from build123d import *

# Parameters (mm, degrees)
EXTRUDE1_DEPTH                                   = 7.9375
CBORE_FOR_1_4_SOCKET_HEAD_CAP_SCREW1_D           = 6.7564
CBORE_FOR_1_4_SOCKET_HEAD_CAP_SCREW1_DEPTH       = 9.525
CBORE_FOR_1_4_SOCKET_HEAD_CAP_SCREW1_CBORE_D     = 11.1125
CBORE_FOR_1_4_SOCKET_HEAD_CAP_SCREW1_CBORE_DEPTH = 6.35
F_1_4_20_TAPPED_HOLE1_D                          = 5.1054
CBORE_FOR_1_4_SOCKET_HEAD_CAP_SCREW2_D           = 6.7564
CBORE_FOR_1_4_SOCKET_HEAD_CAP_SCREW2_DEPTH       = 9.525
CBORE_FOR_1_4_SOCKET_HEAD_CAP_SCREW2_CBORE_D     = 11.1125
CBORE_FOR_1_4_SOCKET_HEAD_CAP_SCREW2_CBORE_DEPTH = 6.35
F_1_4_20_TAPPED_HOLE3_D                          = 5.1054
CBORE_FOR_1_4_SOCKET_HEAD_CAP_SCREW3_D           = 6.7564
CBORE_FOR_1_4_SOCKET_HEAD_CAP_SCREW3_DEPTH       = 9.525
CBORE_FOR_1_4_SOCKET_HEAD_CAP_SCREW3_CBORE_D     = 11.1125
CBORE_FOR_1_4_SOCKET_HEAD_CAP_SCREW3_CBORE_DEPTH = 6.35
F_1_4_20_TAPPED_HOLE4_D                          = 5.1054
FILLET1_R                                        = 3.175


with BuildPart() as part:
    # Sketch1 → Extrude1 (new, symmetric)
    with BuildSketch(Plane.XY):
        with BuildLine():
            Line((-39.6875, 82.55), (-39.6875, 0))
            ThreePointArc((-39.6875, 0), (-32.485618813, -22.798733003), (-13.49375, -37.323134477))
            Line((-13.49375, -37.323134477), (-13.49375, -56.373134477))
            Line((-13.49375, -56.373134477), (-3.96875, -56.373134477))
            Line((-3.96875, -56.373134477), (-3.96875, -36.296166184))
            ThreePointArc((-3.96875, -36.296166184), (0, 36.5125), (3.96875, -36.296166184))
            Line((3.96875, -36.296166184), (3.96875, -56.373134477))
            Line((3.96875, -56.373134477), (13.49375, -56.373134477))
            Line((13.49375, -56.373134477), (13.49375, -37.323134477))
            ThreePointArc((13.49375, -37.323134477), (32.485618813, -22.798733003), (39.6875, 0))
            Line((39.6875, 0), (39.6875, 31.75))
            Line((39.6875, 31.75), (58.7375, 31.75))
            Line((58.7375, 31.75), (58.7375, 41.275))
            Line((58.7375, 41.275), (-30.95625, 41.275))
            ThreePointArc((-30.95625, 41.275), (-34.925, 45.24375), (-30.95625, 49.2125))
            Line((-30.95625, 49.2125), (58.7375, 49.2125))
            Line((58.7375, 49.2125), (58.7375, 58.7375))
            Line((58.7375, 58.7375), (39.6875, 58.7375))
            Line((39.6875, 58.7375), (39.6875, 82.55))
            ThreePointArc((39.6875, 82.55), (32.485618813, 105.348733003), (13.49375, 119.873134477))
            Line((13.49375, 119.873134477), (13.49375, 138.923134477))
            Line((13.49375, 138.923134477), (3.96875, 138.923134477))
            Line((3.96875, 138.923134477), (3.96875, 110.719801693))
            ThreePointArc((3.96875, 110.719801693), (0, 54.102), (-3.96875, 110.719801693))
            Line((-3.96875, 110.719801693), (-3.96875, 138.923134477))
            Line((-3.96875, 138.923134477), (-13.49375, 138.923134477))
            Line((-13.49375, 138.923134477), (-13.49375, 119.873134477))
            ThreePointArc((-13.49375, 119.873134477), (-32.485618813, 105.348733003), (-39.6875, 82.55))
        make_face()
    extrude(amount=EXTRUDE1_DEPTH, both=True)

    # CBORE for 1/4 Socket Head Cap Screw1
    with Locations(Plane(origin=(13.49375, 0, 0), x_dir=(0, 0, -1), z_dir=(1, 0, 0))):
        with Locations((0, 129.398134477)):
            CounterBoreHole(CBORE_FOR_1_4_SOCKET_HEAD_CAP_SCREW1_D / 2, CBORE_FOR_1_4_SOCKET_HEAD_CAP_SCREW1_CBORE_D / 2, CBORE_FOR_1_4_SOCKET_HEAD_CAP_SCREW1_CBORE_DEPTH, depth=CBORE_FOR_1_4_SOCKET_HEAD_CAP_SCREW1_DEPTH)

    # 1/4-20 Tapped Hole1 (through all)
    with Locations(Plane(origin=(-3.96875, 0, 0), x_dir=(0, 0, -1), z_dir=(1, 0, 0))):
        with Locations((0, 129.398134477)):
            Hole(F_1_4_20_TAPPED_HOLE1_D / 2)

    # CBORE for 1/4 Socket Head Cap Screw2
    with Locations(Plane(origin=(0, 58.7375, 0), x_dir=(0, 0, -1), z_dir=(0, 1, 0))):
        with Locations((0, -49.2125)):
            CounterBoreHole(CBORE_FOR_1_4_SOCKET_HEAD_CAP_SCREW2_D / 2, CBORE_FOR_1_4_SOCKET_HEAD_CAP_SCREW2_CBORE_D / 2, CBORE_FOR_1_4_SOCKET_HEAD_CAP_SCREW2_CBORE_DEPTH, depth=CBORE_FOR_1_4_SOCKET_HEAD_CAP_SCREW2_DEPTH)

    # 1/4-20 Tapped Hole3 (through all)
    with Locations(Plane(origin=(0, 41.275, 0), x_dir=(-1, 0, 0), z_dir=(0, 1, 0))):
        with Locations((-49.2125, 0)):
            Hole(F_1_4_20_TAPPED_HOLE3_D / 2)

    # CBORE for 1/4 Socket Head Cap Screw3
    with Locations(Plane(origin=(13.49375, 0, 0), x_dir=(0, 0, -1), z_dir=(1, 0, 0))):
        with Locations((0, -46.848134477)):
            CounterBoreHole(CBORE_FOR_1_4_SOCKET_HEAD_CAP_SCREW3_D / 2, CBORE_FOR_1_4_SOCKET_HEAD_CAP_SCREW3_CBORE_D / 2, CBORE_FOR_1_4_SOCKET_HEAD_CAP_SCREW3_CBORE_DEPTH, depth=CBORE_FOR_1_4_SOCKET_HEAD_CAP_SCREW3_DEPTH)

    # 1/4-20 Tapped Hole4 (through all)
    with Locations(Plane(origin=(-3.96875, 0, 0), x_dir=(0, 0, -1), z_dir=(1, 0, 0))):
        with Locations((0, -46.848134477)):
            Hole(F_1_4_20_TAPPED_HOLE4_D / 2)

    # Fillet1
    fillet1_edges = [part.edges().sort_by_distance(p)[0] for p in [
        (39.6875, 31.75, 0),
        (13.49375, -37.323134477, 0),
        (-13.49375, -37.323134477, 0),
        (-13.49375, 119.873134477, 0),
        (13.49375, 119.873134477, 0),
        (39.6875, 58.7375, 0),
    ]]
    fillet(fillet1_edges, radius=FILLET1_R)


solid = part.part
Input: part model. Units: mm. Frame: model coordinates. A direction names the side the tool comes from. Give positions to 0.01 mm unless a question says otherwise; leave off trailing zeros. Order: outer loops, then holes, each group sorted by start corner. A loop starts at its lowest first (then second) coordinate and runs counter-clockwise, first axis right, second up.
Q1. Section C-C on y = 45.5. Output: boundary loops of the cut face in (x, z), and give its area (3 significant figures).
Checked values:
outline: (-39.69, -7.94) - (-34.92, -7.94) - (-34.92, 7.94) - (-39.69, 7.94) - close
area: 75.7 mm2
Q2. Contact query for flat-ended pins moving along their axis: pin 1 Ø9 at (x, z) = (51.5, -1.5) entering from +Y; pin 2 Ø6.5 at (y, z) = (129.4, 0) entering from +X; pin 3 Ø6 at (y, z) = (98.5, 0) entering from -X. Output: stop coordinate, or through.
Checked values:
pin 1: stops at y = 58.74
pin 2: stops at x = -3.97
pin 3: stops at x = -37.52
Q3. Ray query, probe 1 along X at (y, z) = (-39, 3.75); probe 2 along X at (y, z) = (127, 3); probe 3 along Y at (x, z) = (-8, 6.75) (1 decimal). Return the intervals inside material, ascending.
Checked values:
probe 1: x = -13.53 to -3.97, 3.97 to 13.53
probe 2: x = -13.49 to -3.97, 3.97 to 7.14
probe 3: y = -56.4 to -35.6, 35.6 to 41.3, 49.2 to 55.3, 109.8 to 138.9
Q4. Draft query along Y for faces 6 (the cylindrical face through (5.534, 132.748, -0.44)), 7 (the flat face through (9, -56.373, 0)), 8 (the flat face through (-13, 56, -7.938)), 9 (the flat face through (54, 58.738, 4)). Return one class per face: +Y half, -Y half, draft (parallel to the pull), parting line (faces both ways), or undercut.
Checked values:
face 6: undercut
face 7: -Y half
face 8: draft
face 9: +Y half
Q5. Set-up query: faces 1 (the flat face through (7.144, 125.8, 0.1)), 2 (the flat face through (49, 52.387, -4)), 3 (the flat face through (-3.969, 125, 0)), 4 (the flat face through (3.969, -46, 4)), 5 (the flat face through (39.688, 14, 0)). Return all of +Z, -Z, +X, -X, +Y, -Y with unobstructed straight access to the full face (end or side cutting, diameter ignored); none if empty.
Checked values:
face 1: +X
face 2: +Y
face 3: +Z, -Z, +Y
face 4: +Z, -Z, -Y
face 5: +Z, -Z, +X, -Y
Q6. Section A-A on x = 0. Output: boundary loops of the cut face in (y, z) (1 decimal), and give its area (3 significant figures).
Checked values:
outline: (36.5, -7.9) - (41.3, -7.9) - (41.3, 7.9) - (36.5, 7.9) - close; (49.2, -7.9) - (54.1, -7.9) - (54.1, 7.9) - (49.2, 7.9) - close
area: 153 mm2
Q7. Section B-B on y = 78. Output: boundary loops of the cut face in (x, z), and give its area (3 significant figures).
Checked values:
outline: (-39.69, -7.94) - (-28.08, -7.94) - (-28.08, 7.94) - (-39.69, 7.94) - close; (28.08, -7.94) - (39.69, -7.94) - (39.69, 7.94) - (28.08, 7.94) - close
area: 368 mm2
